Check sheet for the modelled part. Datum: model origin and axes. Units: mm. Coordinates: 2 decimals unless noted, no trailing zeros. Loops run counter-clockwise (first coordinate to the right, second up) from the corner with the lowest first, then second, coordinate; pieces in that order, holes last.
```python
from build123d import *

# Parameters (mm, degrees)
SKETCH_W        = 160
SKETCH_H        = 370
PAD_DEPTH       = 18
POCKET_DEPTH    = 12
CHAMFER_SIZE    = 15
CHAMFER001_SIZE = 15
CHAMFER002_SIZE = 15
FILLET_R        = 5


with BuildPart() as part:
    # Sketch → Pad (new body)
    with BuildSketch(Plane.XY):
        Rectangle(SKETCH_W, SKETCH_H)
    extrude(amount=PAD_DEPTH)

    # Sketch001 → Pocket (cut)
    with BuildSketch(Plane.XY.offset(18)):
        with BuildLine():
            Line((-30, 120), (30, 120))
            ThreePointArc((30, 114), (33, 117), (30, 120))
            Line((30, 114), (30, 108))
            ThreePointArc((30, 102), (33, 105), (30, 108))
            Line((30, 102), (-30, 102))
            ThreePointArc((-30, 108), (-33, 105), (-30, 102))
            Line((-30, 108), (-30, 114))
            ThreePointArc((-30, 120), (-33, 117), (-30, 114))
        make_face()
    pocket = extrude(amount=-POCKET_DEPTH, mode=Mode.SUBTRACT)

    # Mirrored: Pocket across Sketch001 H_Axis
    add(pocket.mirror(Plane(origin=(0, 0, 18), x_dir=(0, 0, 1), z_dir=(0, 1, 0))), mode=Mode.SUBTRACT)

    # Chamfer
    chamfer_edges = [part.edges().sort_by_distance(p)[0] for p in [
        (-80, 185, 9),
    ]]
    chamfer(chamfer_edges, length=CHAMFER_SIZE)

    # Chamfer001
    chamfer001_edges = [part.edges().sort_by_distance(p)[0] for p in [
        (80, 185, 9),
        (80, -185, 9),
    ]]
    chamfer(chamfer001_edges, length=CHAMFER001_SIZE)

    # Chamfer002
    chamfer002_edges = [part.edges().sort_by_distance(p)[0] for p in [
        (-80, -185, 9),
    ]]
    chamfer(chamfer002_edges, length=CHAMFER002_SIZE)

    # Fillet
    fillet_edges = [part.edges().sort_by_distance(p)[0] for p in [
        (-80, -170, 9),
        (-65, -185, 9),
        (-80, 170, 9),
        (-65, 185, 9),
        (65, 185, 9),
        (80, 170, 9),
        (80, -170, 9),
        (65, -185, 9),
    ]]
    fillet(fillet_edges, radius=FILLET_R)


solid = part.part
```
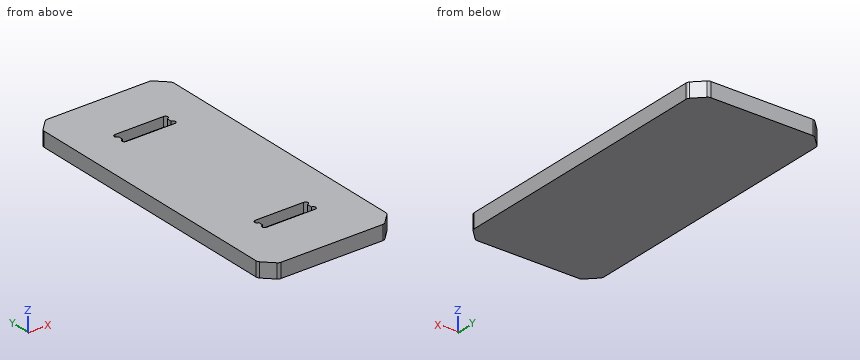
1) Scan lines: line 1 (Y direction, x = 7.5, z = 12); line 2 (Y direction, x = 63, z = 4.25); line 3 (X direction, y = -118.5, z = 10). Record each from-to range of solid material in increasing order.
Answer sheet:
line 1: y = -185 to -120, -102 to 102, 120 to 185
line 2: y = -185 to 185
line 3: x = -80 to -32.6, 32.6 to 80
2) Section check A-A on z = 12. Give the number of separate pieces and of enclosed holes in the cut face, plus the area to 3 significant figures.
Answer sheet:
separate pieces: 1
enclosed holes: 2
area: 56,500 mm2
3) Depth check by flat-ended pin: pin 1 (12 mm diameter, centred on x = -18, y = -109.5, fed in from +Z). Enter the tip coordinate at first touch or a pass-through.
Answer sheet:
pin 1: stops at z = 6
4) Section check B-B on x = 19.5. Enter the section's corners in (y, z), plus the area to 3 significant figures.
Answer sheet:
outline: (-185, 0) - (185, 0) - (185, 18) - (120, 18) - (120, 6) - (102, 6) - (102, 18) - (-102, 18) - (-102, 6) - (-120, 6) - (-120, 18) - (-185, 18) - close
area: 6,230 mm2
